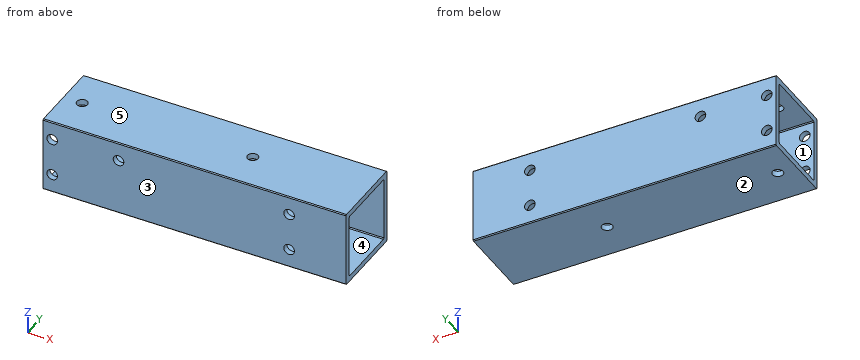
```python
from build123d import *

# Parameters (mm, degrees)
SKETCH1_W                      = 159.85
SKETCH1_H                      = 40
BOSS_EXTRUDE1_DEPTH            = 40
SKETCH2_W                      = 34
SKETCH2_H                      = 34
CUT_EXTRUDE1_DEPTH             = 256.569995305
F_5_6_5_6_DIAMETER_HOLE1_D     = 5.6
F_5_6_5_6_DIAMETER_HOLE1_DEPTH = 3
F_5_6_5_6_DIAMETER_HOLE2_D     = 5.6
F_5_6_5_6_DIAMETER_HOLE2_DEPTH = 3
F_5_6_5_6_DIAMETER_HOLE3_D     = 5.6
F_5_6_5_6_DIAMETER_HOLE4_D     = 5.6
F_5_6_5_6_DIAMETER_HOLE4_DEPTH = 40
CHAMFER1_SIZE                  = 0.5


with BuildPart() as part:
    # Sketch1 → Boss-Extrude1 (new body)
    with BuildSketch(Plane(origin=(0, 142, 0), x_dir=(1, 0, 0), z_dir=(0, 1, 0))):
        with Locations((170.075, -120)):
            Rectangle(SKETCH1_W, SKETCH1_H)
    extrude(amount=-BOSS_EXTRUDE1_DEPTH)

    # Sketch2 → Cut-Extrude1 (cut, through all)
    with BuildSketch(Plane.ZY.offset(-90.15)):
        with Locations((120, 122)):
            Rectangle(SKETCH2_W, SKETCH2_H)
    extrude(amount=-CUT_EXTRUDE1_DEPTH, mode=Mode.SUBTRACT)

    # Ø5.6 (5.6) Diameter Hole1
    with Locations(Plane(origin=(0, 105, 0), x_dir=(1, 0, 0), z_dir=(0, 1, 0))):
        with Locations((220, -130), (220, -110), (130, -130), (95, -130), (95, -110)):
            Hole(F_5_6_5_6_DIAMETER_HOLE1_D / 2, depth=F_5_6_5_6_DIAMETER_HOLE1_DEPTH)

    # Ø5.6 (5.6) Diameter Hole2
    with Locations(Plane(origin=(0, 0, 100), x_dir=(-1, 0, 0), z_dir=(0, 0, -1))):
        with Locations((-190, 122), (-100, 122)):
            Hole(F_5_6_5_6_DIAMETER_HOLE2_D / 2, depth=F_5_6_5_6_DIAMETER_HOLE2_DEPTH)

    # Ø5.6 (5.6) Diameter Hole3 (through all)
    with Locations(Plane(origin=(0, 0, 137), x_dir=(-1, 0, 0), z_dir=(0, 0, -1))):
        with Locations((-190, 122), (-100, 122)):
            Hole(F_5_6_5_6_DIAMETER_HOLE3_D / 2)

    # Ø5.6 (5.6) Diameter Hole4
    with Locations(Plane(origin=(0, 142, 0), x_dir=(1, 0, 0), z_dir=(0, 1, 0))):
        with Locations((220, -130), (220, -110), (130, -130), (95, -130), (95, -110)):
            Hole(F_5_6_5_6_DIAMETER_HOLE4_D / 2, depth=F_5_6_5_6_DIAMETER_HOLE4_DEPTH)

    # Chamfer1
    chamfer1_edges = [part.edges().sort_by_distance(p)[0] for p in [
        (170.075, 102, 100),
        (170.075, 105, 103),
        (170.075, 139, 103),
        (170.075, 139, 137),
        (170.075, 105, 137),
        (170.075, 102, 140),
        (170.075, 142, 100),
        (170.075, 142, 140),
    ]]
    chamfer(chamfer1_edges, length=CHAMFER1_SIZE)


solid = part.part
```
Source: CAD feature listing. Evaluate the final solid. Frame: model axes, mm. Face numbers are marked on the shaded views. A direction names the side the tool comes from. Round coordinates to 2 decimals unless told otherwise and drop trailing zeros. Loops run counter-clockwise (first coordinate to the right, second up) from the corner with the lowest first, then second, coordinate; pieces in that order, holes last. Notation, with made-up numbers: M -20,82 L 18,82 A13 cw 18,100 Z; hole C 73,36 d8. An arc over 180 degrees is marked long. Put each result on its own line as item: value.
(1) Section C-C, the plane x = 147. Return loops of the section in (y, z), and give its area (3 significant figures).
Solutions:
outline: M 102,100.5 L 102.5,100 L 141.5,100 L 142,100.5 L 142,139.5 L 141.5,140 L 102.5,140 L 102,139.5 Z; hole M 105,103.5 L 105.5,103 L 138.5,103 L 139,103.5 L 139,136.5 L 138.5,137 L 105.5,137 L 105,136.5 Z
area: 444 mm²
(2) Section B-B, the plane z = 120. Return loops of the section in (x, y), and give its area (3 significant figures).
Solutions:
outline: M 90.15,102 L 250,102 L 250,105 L 90.15,105 Z; M 90.15,139 L 250,139 L 250,142 L 90.15,142 Z
area: 959 mm²
(3) Ray query, line 1 (Z direction, x = 95, y = 103.25); line 2 (X direction, y = 104, z = 110); line 3 (Z direction, x = 196.5, y = 108.5). Return the intervals inside material, ascending. Write a range as [from, to].
Solutions:
line 1: [100, 107.2], [112.8, 127.2], [132.8, 140]
line 2: [90.15, 92.2], [97.8, 217.2], [222.8, 250]
line 3: [100, 103], [137, 140]
(4) First-contact query: pin 1 (9 mm diameter, centred on x = 190, y = 122, fed in from -Z). Flat tip, straight axial feed; report the tip coordinate or a pass-through.
Solutions:
pin 1: z = 100
(5) Access query for the marked faces 4 and 5. Directions: +Z, -Z, +X, -X, +Y, -Y. A direction counts if a zero-diameter tool reaches every point of the face in a straight line with its end or side. Return the directions, or none.
Solutions:
face 4: +X, -X
face 5: +Z, +X, -X, +Y, -Y
(6) Section D-D, the plane z = 110. Return loops of the section in (x, y).
Solutions:
outline: M 90.15,102 L 92.2,102 L 92.2,105 L 90.15,105 Z; M 90.15,139 L 92.2,139 L 92.2,142 L 90.15,142 Z; M 97.8,102 L 217.2,102 L 217.2,105 L 97.8,105 Z; M 97.8,139 L 217.2,139 L 217.2,142 L 97.8,142 Z; M 222.8,102 L 250,102 L 250,105 L 222.8,105 Z; M 222.8,139 L 250,139 L 250,142 L 222.8,142 Z
(7) Section A-A, the plane y = 127.5. Return loops of the section in (x, z), and give its area (3 significant figures).
Solutions:
outline: M 90.15,100 L 250,100 L 250,103 L 90.15,103 Z; M 90.15,137 L 250,137 L 250,140 L 90.15,140 Z
area: 959 mm²
(8) Pull-direction query (Y, two-part tool) for the marked faces 1, 2 and 3; classes: released by +Y, released by -Y, zero draft, split by the parting line, or undercut.
Solutions:
face 1: undercut
face 2: zero draft
face 3: released by -Y
